Geometry check sheet. Reference: the model listing, model coordinates, mm. Round coordinates to 2 decimals unless told otherwise and drop trailing zeros. Loops run counter-clockwise (first coordinate to the right, second up) from the corner with the lowest first, then second, coordinate; pieces in that order, holes last. Notation, with made-up numbers: M 2,62 L 22,62 A18 ccw 22,79 Z; hole C -3.5,39.25 d2. An arc over 180 degrees is marked long. Write item = value, one per line.
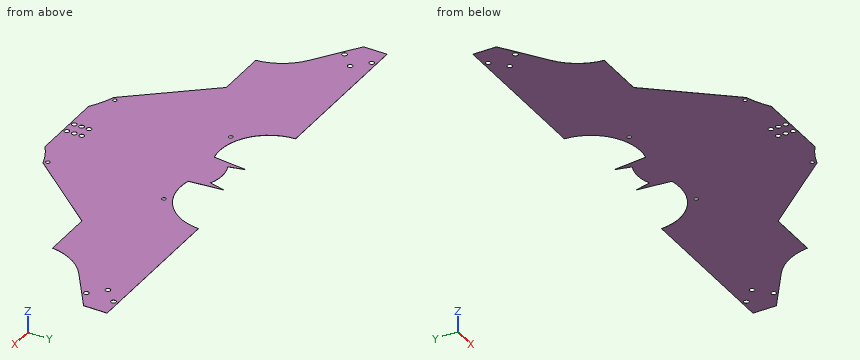
from build123d import *
from OCP.BRepFilletAPI import BRepFilletAPI_MakeChamfer

# Parameters (mm, degrees)
SKETCH2_R           = 1.5875
BOSS_EXTRUDE1_DEPTH = 0.118
SKETCH3_R           = 2
CUT_EXTRUDE1_DEPTH  = 267.27056526
CHAMFER1_SIZE       = 27
CHAMFER1_SIZE2      = 32.960913897
SKETCH4_W           = 60
SKETCH4_H           = 115.138092234
CUT_EXTRUDE2_DEPTH  = 245.436114198
SKETCH5_R           = 2
CUT_EXTRUDE3_DEPTH  = 214.991810964
LPATTERN1_COUNT     = 3
LPATTERN1_PITCH     = 6


with BuildPart() as part:
    # Sketch2 → Boss-Extrude1 (new body)
    with BuildSketch(Plane.XY):
        with BuildLine():
            Line((99.563224144, -21.926473835), (48.69, -83.15))
            ThreePointArc((48.69, -83.15), (13.462751156, -108.648946204), (0, -150))
            ThreePointArc((0, -150), (-13.462751156, -108.648946204), (-48.69, -83.15))
            Line((-48.69, -83.15), (-99.563224144, -21.926473835))
            Line((-99.563224144, -21.926473835), (-140, -21.926473835))
            ThreePointArc((-140, -21.926473835), (-145.965681261, -3.736597624), (-158.952536164, 10.327631798))
            Line((-158.952536164, 10.327631798), (-220, 53.073526165))
            Line((-220, 53.073526165), (-67, 53.073526165))
            ThreePointArc((-67, 53.073526165), (-51.137889855, 23.094319589), (-17.95554779, 16.073526165))
            Line((-17.95554779, 16.073526165), (-15.117733438, 43.073526165))
            Line((-15.117733438, 43.073526165), (-12, 30.568980335))
            ThreePointArc((-12, 30.568980335), (0, 33.073526165), (12, 30.568980335))
            Line((12, 30.568980335), (15.117733438, 43.073526165))
            Line((15.117733438, 43.073526165), (17.95554779, 16.073526165))
            ThreePointArc((17.95554779, 16.073526165), (51.137889855, 23.094319589), (67, 53.073526165))
            Line((67, 53.073526165), (220, 53.073526165))
            Line((220, 53.073526165), (158.952536164, 10.327631798))
            ThreePointArc((158.952536164, 10.327631798), (145.965681261, -3.736597624), (140, -21.926473835))
            Line((140, -21.926473835), (99.563224144, -21.926473835))
        make_face()
        with Locations((46.19, 13)):
            Circle(SKETCH2_R, mode=Mode.SUBTRACT)
        with Locations((-46.19, 13)):
            Circle(SKETCH2_R, mode=Mode.SUBTRACT)
        with Locations((46.19, -80.65)):
            Circle(SKETCH2_R, mode=Mode.SUBTRACT)
        with Locations((-46.19, -80.65)):
            Circle(SKETCH2_R, mode=Mode.SUBTRACT)
    extrude(amount=BOSS_EXTRUDE1_DEPTH)

    # Sketch3 → Cut-Extrude1 (cut, through all)
    with BuildSketch(Plane(origin=(0, 0, 0), x_dir=(-1, 0, 0), z_dir=(0, 0, -1))):
        with Locations((178, 49.573526165)):
            Circle(SKETCH3_R)
        with Locations((178, 27.573526165)):
            Circle(SKETCH3_R)
        with Locations((167, 38.573526165)):
            Circle(SKETCH3_R)
    cut_extrude1 = extrude(amount=-CUT_EXTRUDE1_DEPTH, mode=Mode.SUBTRACT)

    # Mirror2: Cut-Extrude1 across plane
    add(cut_extrude1.mirror(Plane(origin=(0, 0, 0), x_dir=(0, 0, 1), z_dir=(1, 0, 0))), mode=Mode.SUBTRACT)

    # Chamfer1: one chamfer whose edges measure the first distance from different faces: ONE call of the kernel's chamfer builder (chamfer() names one face for all edges)
    chamfer1_edges_1 = [part.edges().sort_by_distance(p)[0] for p in [
        (220, 53.073526165, 0.059),
    ]]
    chamfer1_side_1 = [part.faces().sort_by_distance(p)[0] for p in [
        (143.5, 53.073526165, 0.059),
    ]]
    chamfer1_edges_2 = [part.edges().sort_by_distance(p)[0] for p in [
        (-220, 53.073526165, 0.059),
    ]]
    chamfer1_side_2 = [part.faces().sort_by_distance(p)[0] for p in [
        (-143.5, 53.073526165, 0.059),
    ]]
    chamfer1 = BRepFilletAPI_MakeChamfer(part.part.solid().wrapped)
    for e in chamfer1_edges_1:
        chamfer1.Add(CHAMFER1_SIZE, CHAMFER1_SIZE2, e.wrapped, chamfer1_side_1[0].wrapped)  # the first distance lies on this face
    for e in chamfer1_edges_2:
        chamfer1.Add(CHAMFER1_SIZE, CHAMFER1_SIZE2, e.wrapped, chamfer1_side_2[0].wrapped)  # the first distance lies on this face
    add(Compound.cast(chamfer1.Shape()), mode=Mode.REPLACE)

    # Sketch4 → Cut-Extrude2 (cut, through all)
    with BuildSketch(Plane(origin=(0, 0, 0), x_dir=(-1, 0, 0), z_dir=(0, 0, -1))):
        with Locations((0, -150)):
            Rectangle(SKETCH4_W, SKETCH4_H)
    extrude(amount=-CUT_EXTRUDE2_DEPTH, mode=Mode.SUBTRACT)

    # Sketch5 → Cut-Extrude3 (cut, through all)
    with BuildSketch(Plane(origin=(0, 0, 0), x_dir=(-1, 0, 0), z_dir=(0, 0, -1))):
        with Locations((-5, -89.430953883)):
            Circle(SKETCH5_R)
        with Locations((5, -89.430953883)):
            Circle(SKETCH5_R)
    cut_extrude3 = extrude(amount=-CUT_EXTRUDE3_DEPTH, mode=Mode.SUBTRACT)

    # LPattern1: Cut-Extrude3 ×3
    with Locations(*[(0, i * LPATTERN1_PITCH, 0) for i in range(1, LPATTERN1_COUNT)]):
        add(cut_extrude3, mode=Mode.SUBTRACT)


solid = part.part
(1) Sectioned sample at C-C on y = -59.5. Record the cut outline in (x, z).
Result set:
outline = M -68.34,0 L 68.34,0 L 68.34,0.12 L -68.34,0.12 Z
(2) Sectioned sample at A-A on y = 20. Record the cut outline in (x, z).
Result set:
outline = M -172.77,0 L -46.36,0 L -46.36,0.12 L -172.77,0.12 Z; M -17.54,0 L 17.54,0 L 17.54,0.12 L -17.54,0.12 Z; M 46.36,0 L 172.77,0 L 172.77,0.12 L 46.36,0.12 Z
(3) Material ranges on line 1 along Y through (x, z) = (-57, 0.05); line 2 along X through (y, z) = (10, 0.05), recorded low to high. Write a range as from..to.
Result set:
line_1 = -73.15..28.51
line_2 = -158.49..158.49
(4) Sectioned sample at B-B on x = 125.5. Record the cut outline in (y, z).
Result set:
outline = M -21.93,0 L 53.07,0 L 53.07,0.12 L -21.93,0.12 Z
